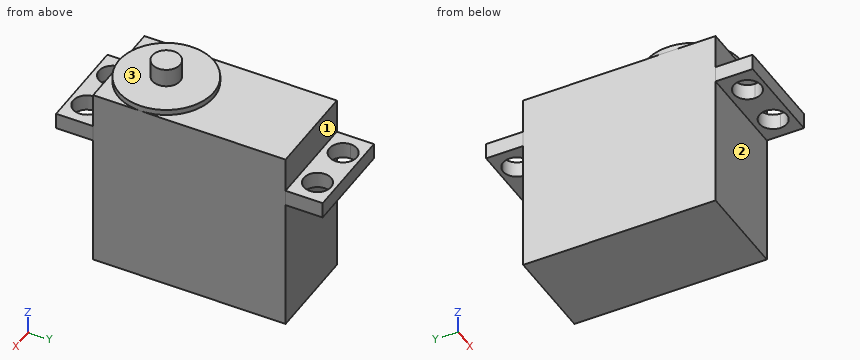
from build123d import *

# Parameters (mm, degrees)
EXTRUDE_1_DEPTH     = 39.1
SKETCH_7_R          = 10.05
EXTRUDE_2_DEPTH     = 1.2
SKETCH_9_R          = 2.95
EXTRUDE_3_DEPTH     = 3.9
SKETCH_10_W         = 20.1
SKETCH_10_H         = 3.4
EXTRUDE_4_DEPTH     = 7.85
SKETCH_11_W         = 20.1
SKETCH_11_H         = 3.4
EXTRUDE_5_DEPTH     = 7.85
CUT_EXTRUDE_1_REACH = 45.602
CUT_EXTRUDE_2_REACH = 45.602


with BuildPart() as part:
    # Sketch 3D_2 → 凸台-拉伸1 (new body)
    with BuildSketch(Plane(origin=(-10.05, 20.35, 0), x_dir=(0.4428021776174894, -0.8966193347777024, 0), z_dir=(0, 0, 1))):
        Polygon((0, 0), (8.90032377, 18.022048629), (45.392730696, 0), (36.492406925, -18.022048629), align=None)
    extrude(amount=-EXTRUDE_1_DEPTH)

    # 草图7 → 凸台-拉伸2 (add)
    with BuildSketch(Plane.XY):
        with Locations((0, -10.3)):
            Circle(SKETCH_7_R)
    extrude(amount=EXTRUDE_2_DEPTH)

    # 草图9 → 凸台-拉伸3 (add)
    with BuildSketch(Plane.XY.offset(1.2)):
        with Locations((0, -10.3)):
            Circle(SKETCH_9_R)
    extrude(amount=EXTRUDE_3_DEPTH)

    # 草图10 → 凸台-拉伸4 (add)
    with BuildSketch(Plane.XZ.offset(20.35)):
        with Locations((0, -9.1)):
            Rectangle(SKETCH_10_W, SKETCH_10_H)
    extrude(amount=EXTRUDE_4_DEPTH)

    # 草图11 → 凸台-拉伸5 (add)
    with BuildSketch(Plane(origin=(0, 20.35, 0), x_dir=(1, 0, 0), z_dir=(0, 1, 0))):
        with Locations((0, 9.1)):
            Rectangle(SKETCH_11_W, SKETCH_11_H)
    extrude(amount=EXTRUDE_5_DEPTH)

    # 草图13 → 切除-拉伸1 (cut, up to next)
    with BuildSketch(Plane.XY.offset(-7.4), mode=Mode.PRIVATE) as cut_extrude_1_sk1:
        with BuildLine():
            ThreePointArc((-7.95, -24.4), (-7.100609665, -26.450609665), (-5.05, -27.3))
            Line((-5.05, -27.3), (-5.05, -24.4))
            Line((-5.05, -24.4), (-7.95, -24.4))
        make_face()
    cut_extrude_1_tool1 = extrude(cut_extrude_1_sk1.sketch, amount=-CUT_EXTRUDE_1_REACH, mode=Mode.PRIVATE) & part.part
    # 草图13 → 切除-拉伸1 (cut, up to next)
    with BuildSketch(Plane.XY.offset(-7.4), mode=Mode.PRIVATE) as cut_extrude_1_sk2:
        with BuildLine():
            Line((-5.05, -24.4), (-5.05, -27.3))
            ThreePointArc((-5.05, -27.3), (-2.999390335, -26.450609665), (-2.15, -24.4))
            ThreePointArc((-2.15, -24.4), (-5.05, -21.5), (-7.95, -24.4))
            Line((-7.95, -24.4), (-5.05, -24.4))
        make_face()
    cut_extrude_1_tool2 = extrude(cut_extrude_1_sk2.sketch, amount=-CUT_EXTRUDE_1_REACH, mode=Mode.PRIVATE) & part.part
    # 草图13 → 切除-拉伸1 (cut, up to next)
    with BuildSketch(Plane.XY.offset(-7.4), mode=Mode.PRIVATE) as cut_extrude_1_sk3:
        with BuildLine():
            ThreePointArc((-7.95, -24.4), (-7.100609665, -26.450609665), (-5.05, -27.3))
            Line((-5.05, -27.3), (-5.05, -24.4))
            Line((-5.05, -24.4), (-7.95, -24.4))
        make_face()
    cut_extrude_1_tool3 = extrude(cut_extrude_1_sk3.sketch, amount=-CUT_EXTRUDE_1_REACH, mode=Mode.PRIVATE) & part.part
    # 草图13 → 切除-拉伸1 (cut, up to next)
    with BuildSketch(Plane.XY.offset(-7.4), mode=Mode.PRIVATE) as cut_extrude_1_sk4:
        with BuildLine():
            Line((-5.05, -24.4), (-5.05, -27.3))
            ThreePointArc((-5.05, -27.3), (-2.999390335, -26.450609665), (-2.15, -24.4))
            ThreePointArc((-2.15, -24.4), (-5.05, -21.5), (-7.95, -24.4))
            Line((-7.95, -24.4), (-5.05, -24.4))
        make_face()
    cut_extrude_1_tool4 = extrude(cut_extrude_1_sk4.sketch, amount=-CUT_EXTRUDE_1_REACH, mode=Mode.PRIVATE) & part.part
    # 草图13 → 切除-拉伸1 (cut, up to next)
    with BuildSketch(Plane.XY.offset(-7.4), mode=Mode.PRIVATE) as cut_extrude_1_sk5:
        with BuildLine():
            ThreePointArc((7.95, -24.4), (2.999390335, -22.349390335), (5.05, -27.3))
            Line((5.05, -27.3), (5.05, -24.4))
            Line((5.05, -24.4), (7.95, -24.4))
        make_face()
    cut_extrude_1_tool5 = extrude(cut_extrude_1_sk5.sketch, amount=-CUT_EXTRUDE_1_REACH, mode=Mode.PRIVATE) & part.part
    # 草图13 → 切除-拉伸1 (cut, up to next)
    with BuildSketch(Plane.XY.offset(-7.4), mode=Mode.PRIVATE) as cut_extrude_1_sk6:
        with BuildLine():
            Line((5.05, -24.4), (5.05, -27.3))
            ThreePointArc((5.05, -27.3), (7.100609665, -26.450609665), (7.95, -24.4))
            Line((7.95, -24.4), (5.05, -24.4))
        make_face()
    cut_extrude_1_tool6 = extrude(cut_extrude_1_sk6.sketch, amount=-CUT_EXTRUDE_1_REACH, mode=Mode.PRIVATE) & part.part
    # 草图13 → 切除-拉伸1 (cut, up to next)
    with BuildSketch(Plane.XY.offset(-7.4), mode=Mode.PRIVATE) as cut_extrude_1_sk7:
        with BuildLine():
            ThreePointArc((7.95, -24.4), (2.999390335, -22.349390335), (5.05, -27.3))
            Line((5.05, -27.3), (5.05, -24.4))
            Line((5.05, -24.4), (7.95, -24.4))
        make_face()
    cut_extrude_1_tool7 = extrude(cut_extrude_1_sk7.sketch, amount=-CUT_EXTRUDE_1_REACH, mode=Mode.PRIVATE) & part.part
    # 草图13 → 切除-拉伸1 (cut, up to next)
    with BuildSketch(Plane.XY.offset(-7.4), mode=Mode.PRIVATE) as cut_extrude_1_sk8:
        with BuildLine():
            Line((5.05, -24.4), (5.05, -27.3))
            ThreePointArc((5.05, -27.3), (7.100609665, -26.450609665), (7.95, -24.4))
            Line((7.95, -24.4), (5.05, -24.4))
        make_face()
    cut_extrude_1_tool8 = extrude(cut_extrude_1_sk8.sketch, amount=-CUT_EXTRUDE_1_REACH, mode=Mode.PRIVATE) & part.part
    add(cut_extrude_1_tool1.solids().sort_by_distance((-6.280798, -25.630798, -7.4))[0], mode=Mode.SUBTRACT)
    add(cut_extrude_1_tool2.solids().sort_by_distance((-4.639734, -23.989734, -7.4))[0], mode=Mode.SUBTRACT)
    add(cut_extrude_1_tool3.solids().sort_by_distance((-6.280798, -25.630798, -7.4))[0], mode=Mode.SUBTRACT)
    add(cut_extrude_1_tool4.solids().sort_by_distance((-4.639734, -23.989734, -7.4))[0], mode=Mode.SUBTRACT)
    add(cut_extrude_1_tool5.solids().sort_by_distance((4.639734, -23.989734, -7.4))[0], mode=Mode.SUBTRACT)
    add(cut_extrude_1_tool6.solids().sort_by_distance((6.280798, -25.630798, -7.4))[0], mode=Mode.SUBTRACT)
    add(cut_extrude_1_tool7.solids().sort_by_distance((4.639734, -23.989734, -7.4))[0], mode=Mode.SUBTRACT)
    add(cut_extrude_1_tool8.solids().sort_by_distance((6.280798, -25.630798, -7.4))[0], mode=Mode.SUBTRACT)

    # 草图14 → 切除-拉伸2 (cut, up to next)
    with BuildSketch(Plane.XY.offset(-7.4), mode=Mode.PRIVATE) as cut_extrude_2_sk1:
        with BuildLine():
            ThreePointArc((-2.15, 24.4), (-2.999390335, 26.450609665), (-5.05, 27.3))
            Line((-5.05, 27.3), (-5.05, 24.4))
            Line((-5.05, 24.4), (-7.95, 24.4))
            ThreePointArc((-7.95, 24.4), (-5.05, 21.5), (-2.15, 24.4))
        make_face()
    cut_extrude_2_tool1 = extrude(cut_extrude_2_sk1.sketch, amount=-CUT_EXTRUDE_2_REACH, mode=Mode.PRIVATE) & part.part
    # 草图14 → 切除-拉伸2 (cut, up to next)
    with BuildSketch(Plane.XY.offset(-7.4), mode=Mode.PRIVATE) as cut_extrude_2_sk2:
        with BuildLine():
            Line((-5.05, 24.4), (-5.05, 27.3))
            ThreePointArc((-5.05, 27.3), (-7.100609665, 26.450609665), (-7.95, 24.4))
            Line((-7.95, 24.4), (-5.05, 24.4))
        make_face()
    cut_extrude_2_tool2 = extrude(cut_extrude_2_sk2.sketch, amount=-CUT_EXTRUDE_2_REACH, mode=Mode.PRIVATE) & part.part
    # 草图14 → 切除-拉伸2 (cut, up to next)
    with BuildSketch(Plane.XY.offset(-7.4), mode=Mode.PRIVATE) as cut_extrude_2_sk3:
        with BuildLine():
            ThreePointArc((-2.15, 24.4), (-2.999390335, 26.450609665), (-5.05, 27.3))
            Line((-5.05, 27.3), (-5.05, 24.4))
            Line((-5.05, 24.4), (-7.95, 24.4))
            ThreePointArc((-7.95, 24.4), (-5.05, 21.5), (-2.15, 24.4))
        make_face()
    cut_extrude_2_tool3 = extrude(cut_extrude_2_sk3.sketch, amount=-CUT_EXTRUDE_2_REACH, mode=Mode.PRIVATE) & part.part
    # 草图14 → 切除-拉伸2 (cut, up to next)
    with BuildSketch(Plane.XY.offset(-7.4), mode=Mode.PRIVATE) as cut_extrude_2_sk4:
        with BuildLine():
            Line((-5.05, 24.4), (-5.05, 27.3))
            ThreePointArc((-5.05, 27.3), (-7.100609665, 26.450609665), (-7.95, 24.4))
            Line((-7.95, 24.4), (-5.05, 24.4))
        make_face()
    cut_extrude_2_tool4 = extrude(cut_extrude_2_sk4.sketch, amount=-CUT_EXTRUDE_2_REACH, mode=Mode.PRIVATE) & part.part
    # 草图14 → 切除-拉伸2 (cut, up to next)
    with BuildSketch(Plane.XY.offset(-7.4), mode=Mode.PRIVATE) as cut_extrude_2_sk5:
        with BuildLine():
            ThreePointArc((7.95, 24.4), (7.100609665, 26.450609665), (5.05, 27.3))
            Line((5.05, 27.3), (5.05, 24.4))
            Line((5.05, 24.4), (7.95, 24.4))
        make_face()
    cut_extrude_2_tool5 = extrude(cut_extrude_2_sk5.sketch, amount=-CUT_EXTRUDE_2_REACH, mode=Mode.PRIVATE) & part.part
    # 草图14 → 切除-拉伸2 (cut, up to next)
    with BuildSketch(Plane.XY.offset(-7.4), mode=Mode.PRIVATE) as cut_extrude_2_sk6:
        with BuildLine():
            Line((5.05, 24.4), (5.05, 27.3))
            ThreePointArc((5.05, 27.3), (2.999390335, 22.349390335), (7.95, 24.4))
            Line((7.95, 24.4), (5.05, 24.4))
        make_face()
    cut_extrude_2_tool6 = extrude(cut_extrude_2_sk6.sketch, amount=-CUT_EXTRUDE_2_REACH, mode=Mode.PRIVATE) & part.part
    # 草图14 → 切除-拉伸2 (cut, up to next)
    with BuildSketch(Plane.XY.offset(-7.4), mode=Mode.PRIVATE) as cut_extrude_2_sk7:
        with BuildLine():
            ThreePointArc((7.95, 24.4), (7.100609665, 26.450609665), (5.05, 27.3))
            Line((5.05, 27.3), (5.05, 24.4))
            Line((5.05, 24.4), (7.95, 24.4))
        make_face()
    cut_extrude_2_tool7 = extrude(cut_extrude_2_sk7.sketch, amount=-CUT_EXTRUDE_2_REACH, mode=Mode.PRIVATE) & part.part
    # 草图14 → 切除-拉伸2 (cut, up to next)
    with BuildSketch(Plane.XY.offset(-7.4), mode=Mode.PRIVATE) as cut_extrude_2_sk8:
        with BuildLine():
            Line((5.05, 24.4), (5.05, 27.3))
            ThreePointArc((5.05, 27.3), (2.999390335, 22.349390335), (7.95, 24.4))
            Line((7.95, 24.4), (5.05, 24.4))
        make_face()
    cut_extrude_2_tool8 = extrude(cut_extrude_2_sk8.sketch, amount=-CUT_EXTRUDE_2_REACH, mode=Mode.PRIVATE) & part.part
    add(cut_extrude_2_tool1.solids().sort_by_distance((-4.639734, 23.989734, -7.4))[0], mode=Mode.SUBTRACT)
    add(cut_extrude_2_tool2.solids().sort_by_distance((-6.280798, 25.630798, -7.4))[0], mode=Mode.SUBTRACT)
    add(cut_extrude_2_tool3.solids().sort_by_distance((-4.639734, 23.989734, -7.4))[0], mode=Mode.SUBTRACT)
    add(cut_extrude_2_tool4.solids().sort_by_distance((-6.280798, 25.630798, -7.4))[0], mode=Mode.SUBTRACT)
    add(cut_extrude_2_tool5.solids().sort_by_distance((6.280798, 25.630798, -7.4))[0], mode=Mode.SUBTRACT)
    add(cut_extrude_2_tool6.solids().sort_by_distance((4.639734, 23.989734, -7.4))[0], mode=Mode.SUBTRACT)
    add(cut_extrude_2_tool7.solids().sort_by_distance((6.280798, 25.630798, -7.4))[0], mode=Mode.SUBTRACT)
    add(cut_extrude_2_tool8.solids().sort_by_distance((4.639734, 23.989734, -7.4))[0], mode=Mode.SUBTRACT)


solid = part.part
The model under review builds one solid part; all positions refer to its coordinate system, in mm. Face numbers are marked on the shaded views. A direction names the side the tool comes from. Round coordinates to 2 decimals unless told otherwise and drop trailing zeros. Loops run counter-clockwise (first coordinate to the right, second up) from the corner with the lowest first, then second, coordinate; pieces in that order, holes last. Notation, with made-up numbers: (66.25, -39.75) -> (121.25, -39.75) arc R37 ccw to (121.25, -0.75) -> close; hole circle Ø2 at (3, -28). An arc over 180 degrees is marked (long way). Write item = value, one per line. Start each with the question number.
Item 1: Take a section at A-A on z = -8. Give the boundary of the cut face in (x, y).
Item 2: Take a section at D-D on z = -18. Give the boundary of the cut face in (x, y), plus the area to 3 significant figures.
Item 3: Insertion check: pin 1 (6 mm diameter, centred on x = 0.5, z = -2.5, fed in from -Y); pin 2 (11 mm diameter, centred on x = -7, y = -16, fed in from +Z); pin 3 (5 mm diameter, centred on x = 3, y = 16.5, fed in from +Z); pin 4 (3.5 mm diameter, centred on x = 5.05, y = 24.4, fed in from -Z). Each pin has a flat end and moves straight along its axis. Give the tip position at first contact, or say it passes through.
Item 4: Take a section at B-B on x = -6.5. Give the boundary of the cut face in (y, z).
Item 5: Take a section at C-C on y = 22.5. Give the boundary of the cut face in (x, z), plus the area to 3 significant figures.
Item 6: For the marked faces 1, 2 and 3, list the 3-axis set-ups (+Z, -Z, +X, -X, +Y, -Y) from which the entire face can be reached by the end or side of a thin tool; tool diameter is ignored.
Item 7: To check wall thickness, follow L1, parallel to Y at x = 5.05, z = -9.6; L2, parallel to X at y = 24.4, z = -9.25; L3, parallel to Y at x = 7.75, z = -19. State the ranges of each line that lie inside material, in increasing order.
Result:
q1.outline = (-10.05, -28.2) -> (10.05, -28.2) -> (10.05, 28.2) -> (-10.05, 28.2) -> close; hole circle Ø5.8 at (-5.05, -24.4); hole circle Ø5.8 at (-5.05, 24.4); hole circle Ø5.8 at (5.05, -24.4); hole circle Ø5.8 at (5.05, 24.4)
q2.outline = (-10.05, -20.35) -> (10.05, -20.35) -> (10.05, 20.35) -> (-10.05, 20.35) -> close
q2.area = 818 mm²
q3.pin_1 = -20.35
q3.pin_2 = 1.2
q3.pin_3 = 0
q3.pin_4 = through
q4.outline = (-28.2, -10.8) -> (-26.91, -10.8) -> (-26.91, -7.4) -> (-28.2, -7.4) -> close; (-21.89, -10.8) -> (-20.35, -10.8) -> (-20.35, -39.1) -> (20.35, -39.1) -> (20.35, -10.8) -> (21.89, -10.8) -> (21.89, -7.4) -> (20.35, -7.4) -> (20.35, 0) -> (-2.63, 0) -> (-2.63, 1.2) -> (-17.97, 1.2) -> (-17.97, 0) -> (-20.35, 0) -> (-20.35, -7.4) -> (-21.89, -7.4) -> close; (26.91, -10.8) -> (28.2, -10.8) -> (28.2, -7.4) -> (26.91, -7.4) -> close
q5.outline = (-10.05, -10.8) -> (-7.24, -10.8) -> (-7.24, -7.4) -> (-10.05, -7.4) -> close; (-2.86, -10.8) -> (2.86, -10.8) -> (2.86, -7.4) -> (-2.86, -7.4) -> close; (7.24, -10.8) -> (10.05, -10.8) -> (10.05, -7.4) -> (7.24, -7.4) -> close
q5.area = 38.5 mm²
q6.face_1 = +Z, +X, -X, +Y
q6.face_2 = -Z, +X, -X, -Y
q6.face_3 = +Z
q7.L1 = -28.2 to -27.3, -21.5 to 21.5, 27.3 to 28.2
q7.L2 = -10.05 to -7.95, -2.15 to 2.15, 7.95 to 10.05
q7.L3 = -20.35 to 20.35
